```python
from build123d import *

# Parameters (mm, degrees)
SKETCH_1_W                = 83
SKETCH_1_H                = 127
EXTRUDE_1_DEPTH           = 36
SKETCH_2_W                = 77
SKETCH_2_H                = 40.7
CUT_EXTRUDE_1_DEPTH       = 22.9
SKETCH_3_W                = 77
SKETCH_3_H                = 78
CUT_EXTRUDE_4_DEPTH       = 33
SKETCH_4_W                = 31.5
SKETCH_4_H                = 25.3
EXTRUDE_2_DEPTH           = 11
SKETCH_5_W                = 25.5
SKETCH_5_H                = 23.3
CUT_EXTRUDE_5_DEPTH       = 11
CUT_EXTRUDE_6_DEPTH       = 14
CUT_EXTRUDE_6_DEPTH_BACK  = 10
SKETCH_6_R                = 1.5
SKETCH_7_R                = 2.5
CUT_EXTRUDE_7_DEPTH       = 22
CUT_EXTRUDE_8_DEPTH       = 23
CUT_EXTRUDE_8_DEPTH_BACK  = 30
SKETCH_8_R                = 2.7
CUT_EXTRUDE_9_DEPTH       = 11
CUT_EXTRUDE_9_DEPTH_BACK  = 33
SKETCH_9_W                = 12
SKETCH_9_H                = 10.9
CUT_EXTRUDE_10_DEPTH      = 14
CUT_EXTRUDE_10_DEPTH_BACK = 36
SKETCH_10_W               = 9
SKETCH_10_H               = 10.5
SKETCH_11_W               = 78
SKETCH_11_H               = 3
EXTRUDE_3_DEPTH           = 4
SKETCH_12_W               = 69
SKETCH_12_H               = 3
EXTRUDE_4_DEPTH           = 4
SKETCH_13_W               = 78
SKETCH_13_H               = 3
EXTRUDE_5_DEPTH           = 4
SKETCH_15_W               = 69
SKETCH_15_H               = 3
EXTRUDE_6_DEPTH           = 2
SKETCH_16_W               = 1.5
SKETCH_16_H               = 41.5
CUT_EXTRUDE_11_DEPTH      = 2
SKETCH_17_W               = 78.5
SKETCH_17_H               = 1.5
CUT_EXTRUDE_12_DEPTH      = 2
SKETCH_19_W               = 1.5
SKETCH_19_H               = 42.211102857
CUT_EXTRUDE_13_DEPTH      = 2
FILLET_1_R                = 2
FILLET_2_R                = 2
FILLET_3_R                = 2
FILLET_4_R                = 2
FILLET_5_R                = 2
SKETCH_20_W               = 8
SKETCH_20_H               = 10
CUT_EXTRUDE_14_DEPTH      = 2
SKETCH_21_W               = 8
SKETCH_21_H               = 10
CUT_EXTRUDE_15_DEPTH      = 2
CUT_EXTRUDE_16_DEPTH      = 102
CUT_EXTRUDE_16_DEPTH_BACK = 85
SKETCH_22_R               = 1.5
CUT_EXTRUDE_17_DEPTH      = 37
CUT_EXTRUDE_17_DEPTH_BACK = 68
SKETCH_23_R               = 1.5


with BuildPart() as part:
    # Эскиз1 → Бобышка-Вытянуть1 (new body)
    with BuildSketch(Plane(origin=(0, 0, 0), x_dir=(1, 0, 0), z_dir=(0, 1, 0))):
        with Locations((-41.5, 63.5)):
            Rectangle(SKETCH_1_W, SKETCH_1_H)
    extrude(amount=EXTRUDE_1_DEPTH)

    # Эскиз2 → Вырез-Вытянуть1 (cut)
    with BuildSketch(Plane(origin=(0, 0, 0), x_dir=(-1, 0, 0), z_dir=(0, -1, 0))):
        with Locations((41.5, 23.35)):
            Rectangle(SKETCH_2_W, SKETCH_2_H)
    extrude(amount=-CUT_EXTRUDE_1_DEPTH, mode=Mode.SUBTRACT)

    # Эскиз3 → Вырез-Вытянуть4 (cut)
    with BuildSketch(Plane(origin=(0, 36, 0), x_dir=(1, 0, 0), z_dir=(0, 1, 0))):
        with Locations((-41.5, 85)):
            Rectangle(SKETCH_3_W, SKETCH_3_H)
    extrude(amount=-CUT_EXTRUDE_4_DEPTH, mode=Mode.SUBTRACT)

    # Эскиз4 → Бобышка-Вытянуть2 (add)
    with BuildSketch(Plane(origin=(0, 3, 0), x_dir=(1, 0, 0), z_dir=(0, 1, 0))):
        with Locations((-41.5, 58.65)):
            Rectangle(SKETCH_4_W, SKETCH_4_H)
    extrude(amount=EXTRUDE_2_DEPTH)

    # Эскиз5 → Вырез-Вытянуть5 (cut)
    with BuildSketch(Plane(origin=(0, 14, 0), x_dir=(1, 0, 0), z_dir=(0, 1, 0))):
        with Locations((-41.5, 59.65)):
            Rectangle(SKETCH_5_W, SKETCH_5_H)
    extrude(amount=-CUT_EXTRUDE_5_DEPTH, mode=Mode.SUBTRACT)

    # Эскиз6 → Вырез-Вытянуть6 (cut, two sides: drawn at the far end of the back side and taken through both)
    with BuildSketch(Plane(origin=(0, 0, 0), x_dir=(0, 0, -1), z_dir=(1, 0, 0)).offset(-CUT_EXTRUDE_6_DEPTH_BACK)):
        with Locations(Location((60.742856383, 18, 0), (0, 0, 180))):
            Circle(SKETCH_6_R)
    extrude(amount=CUT_EXTRUDE_6_DEPTH + CUT_EXTRUDE_6_DEPTH_BACK, mode=Mode.SUBTRACT)

    # Эскиз7 → Вырез-Вытянуть7 (cut)
    with BuildSketch(Plane.XY.offset(-43.7)):
        with Locations((-5.5, 19.4)):
            Circle(SKETCH_7_R)
    extrude(amount=-CUT_EXTRUDE_7_DEPTH, mode=Mode.SUBTRACT)

    # Эскиз8 → Вырез-Вытянуть8 (cut, two sides: drawn at the far end of the back side and taken through both)
    with BuildSketch(Plane(origin=(0, 0, -127), x_dir=(-1, 0, 0), z_dir=(0, 0, -1)).offset(-CUT_EXTRUDE_8_DEPTH_BACK)):
        with Locations(Location((72.842031124, 26.425424665, 0), (0, 0, 180))):
            Circle(SKETCH_8_R)
    extrude(amount=CUT_EXTRUDE_8_DEPTH + CUT_EXTRUDE_8_DEPTH_BACK, mode=Mode.SUBTRACT)

    # Эскиз9 → Вырез-Вытянуть9 (cut, two sides: drawn at the far end of the back side and taken through both)
    with BuildSketch(Plane.ZY.offset(3).offset(-CUT_EXTRUDE_9_DEPTH_BACK)):
        with Locations((-87, 9.65)):
            Rectangle(SKETCH_9_W, SKETCH_9_H)
    extrude(amount=CUT_EXTRUDE_9_DEPTH + CUT_EXTRUDE_9_DEPTH_BACK, mode=Mode.SUBTRACT)

    # Эскиз10 → Вырез-Вытянуть10 (cut, two sides: drawn at the far end of the back side and taken through both)
    with BuildSketch(Plane.ZY.offset(3).offset(-CUT_EXTRUDE_10_DEPTH_BACK)):
        with Locations((-116.5, 9.35)):
            Rectangle(SKETCH_10_W, SKETCH_10_H)
    extrude(amount=CUT_EXTRUDE_10_DEPTH + CUT_EXTRUDE_10_DEPTH_BACK, mode=Mode.SUBTRACT)

    # Эскиз11 → Бобышка-Вытянуть3 (add)
    with BuildSketch(Plane.ZY.offset(3)):
        with Locations((-85, 31.5)):
            Rectangle(SKETCH_11_W, SKETCH_11_H)
    extrude(amount=EXTRUDE_3_DEPTH)

    # Эскиз12 → Бобышка-Вытянуть4 (add)
    with BuildSketch(Plane.XY.offset(-124)):
        with Locations((-41.5, 31.5)):
            Rectangle(SKETCH_12_W, SKETCH_12_H)
    extrude(amount=EXTRUDE_4_DEPTH)

    # Эскиз13 → Бобышка-Вытянуть5 (add)
    with BuildSketch(Plane(origin=(-80, 0, 0), x_dir=(0, 0, -1), z_dir=(1, 0, 0))):
        with Locations((85, 31.5)):
            Rectangle(SKETCH_13_W, SKETCH_13_H)
    extrude(amount=EXTRUDE_5_DEPTH)

    # Эскиз15 → Бобышка-Вытянуть6 (add)
    with BuildSketch(Plane(origin=(0, 0, -46), x_dir=(-1, 0, 0), z_dir=(0, 0, -1))):
        with Locations((41.5, 31.5)):
            Rectangle(SKETCH_15_W, SKETCH_15_H)
    extrude(amount=EXTRUDE_6_DEPTH)

    # Эскиз16 → Вырез-Вытянуть11 (cut)
    with BuildSketch(Plane(origin=(0, 0, 0), x_dir=(-1, 0, 0), z_dir=(0, -1, 0))):
        with Locations((2.25, 23.75)):
            Rectangle(SKETCH_16_W, SKETCH_16_H)
    extrude(amount=-CUT_EXTRUDE_11_DEPTH, mode=Mode.SUBTRACT)

    # Эскиз17 → Вырез-Вытянуть12 (cut)
    with BuildSketch(Plane.XZ):
        with Locations((-40.75, -44.45)):
            Rectangle(SKETCH_17_W, SKETCH_17_H)
    extrude(amount=-CUT_EXTRUDE_12_DEPTH, mode=Mode.SUBTRACT)

    # Эскиз19 → Вырез-Вытянуть13 (cut)
    with BuildSketch(Plane.XZ):
        with Locations((-80.75, -24.094448572)):
            Rectangle(SKETCH_19_W, SKETCH_19_H)
    extrude(amount=-CUT_EXTRUDE_13_DEPTH, mode=Mode.SUBTRACT)

    # Скругление1
    fillet_1_edges = [part.edges().sort_by_distance(p)[0] for p in [
        (-41.5, 36, -127),
    ]]
    fillet(fillet_1_edges, radius=FILLET_1_R)

    # Скругление2
    fillet_2_edges = [part.edges().sort_by_distance(p)[0] for p in [
        (-83, 36, -62.5),
        (-83, 17, -127),
        (-83, 35.414213562, -126.414213562),
    ]]
    fillet(fillet_2_edges, radius=FILLET_2_R)

    # Скругление3
    fillet_3_edges = [part.edges().sort_by_distance(p)[0] for p in [
        (-83, 17, 0),
        (-40.5, 36, 0),
        (-82.414213562, 35.414213562, 0),
    ]]
    fillet(fillet_3_edges, radius=FILLET_3_R)

    # Скругление4
    fillet_4_edges = [part.edges().sort_by_distance(p)[0] for p in [
        (0, 17, -127),
        (0, 35.414213562, -126.414213562),
        (0, 17, 0),
        (0, 36, -63.5),
        (0, 35.414213562, -0.585786438),
    ]]
    fillet(fillet_4_edges, radius=FILLET_4_R)

    # Скругление5
    # the kernel refuses this fillet: 2 mm, written as the material it takes off along each edge
    with BuildSketch(Plane(origin=(-2, 0, -125), x_dir=(1, 0, 0), z_dir=(0, 0, 1))) as fillet_5_piece_1:
        with BuildLine():
            CenterArc((2 - FILLET_5_R, FILLET_5_R), FILLET_5_R, 270, 90)
            Line((2, FILLET_5_R), (2, 0))
            Line((2, 0), (2 - FILLET_5_R, 0))
        make_face()
    revolve(axis=Axis((-2, 0, -125), (0, 1, 0)), revolution_arc=90, mode=Mode.SUBTRACT)
    with BuildSketch(Plane(origin=(0, 0, -125), x_dir=(0, 1, 0), z_dir=(0, 0, 1))) as fillet_5_piece_2:
        with BuildLine():
            CenterArc((FILLET_5_R, FILLET_5_R), FILLET_5_R, 180, 90)
            Line((0, FILLET_5_R), (0, 0))
            Line((0, 0), (FILLET_5_R, 0))
        make_face()
    extrude(amount=123, mode=Mode.SUBTRACT)
    with BuildSketch(Plane(origin=(-2, 0, -2), x_dir=(1, 0, 0), z_dir=(0, 0, -1))) as fillet_5_piece_3:
        with BuildLine():
            CenterArc((2 - FILLET_5_R, -FILLET_5_R), FILLET_5_R, 0, 90)
            Line((2, -FILLET_5_R), (2, 0))
            Line((2, 0), (2 - FILLET_5_R, 0))
        make_face()
    revolve(axis=Axis((-2, 0, -2), (0, -1, 0)), revolution_arc=90, mode=Mode.SUBTRACT)
    with BuildSketch(Plane(origin=(-2, 0, 0), x_dir=(0, 0, -1), z_dir=(-1, 0, 0)), Plane(origin=(-81, 0, -127), x_dir=(0, 0, 1), z_dir=(1, 0, 0))) as fillet_5_piece_4:
        with BuildLine():
            CenterArc((FILLET_5_R, -FILLET_5_R), FILLET_5_R, 90, 90)
            Line((0, -FILLET_5_R), (0, 0))
            Line((0, 0), (FILLET_5_R, 0))
        make_face()
    extrude(amount=79, mode=Mode.SUBTRACT)
    with BuildSketch(Plane(origin=(-81, 0, -2), x_dir=(-1, 0, 0), z_dir=(0, 0, -1))) as fillet_5_piece_5:
        with BuildLine():
            CenterArc((2 - FILLET_5_R, FILLET_5_R), FILLET_5_R, 270, 90)
            Line((2, FILLET_5_R), (2, 0))
            Line((2, 0), (2 - FILLET_5_R, 0))
        make_face()
    revolve(axis=Axis((-81, 0, -2), (0, 1, 0)), revolution_arc=90, mode=Mode.SUBTRACT)
    with BuildSketch(Plane(origin=(-83, 0, -2), x_dir=(1, 0, 0), z_dir=(0, 0, -1))) as fillet_5_piece_6:
        with BuildLine():
            CenterArc((FILLET_5_R, -FILLET_5_R), FILLET_5_R, 90, 90)
            Line((0, -FILLET_5_R), (0, 0))
            Line((0, 0), (FILLET_5_R, 0))
        make_face()
    extrude(amount=123, mode=Mode.SUBTRACT)
    with BuildSketch(Plane(origin=(-81, 0, -125), x_dir=(-1, 0, 0), z_dir=(0, 0, 1))) as fillet_5_piece_7:
        with BuildLine():
            CenterArc((2 - FILLET_5_R, -FILLET_5_R), FILLET_5_R, 0, 90)
            Line((2, -FILLET_5_R), (2, 0))
            Line((2, 0), (2 - FILLET_5_R, 0))
        make_face()
    revolve(axis=Axis((-81, 0, -125), (0, -1, 0)), revolution_arc=90, mode=Mode.SUBTRACT)

    # Эскиз20 → Вырез-Вытянуть14 (cut)
    with BuildSketch(Plane.XZ):
        with Locations((-15, -50.2)):
            Rectangle(SKETCH_20_W, SKETCH_20_H)
    extrude(amount=-CUT_EXTRUDE_14_DEPTH, mode=Mode.SUBTRACT)

    # Эскиз21 → Вырез-Вытянуть15 (cut)
    with BuildSketch(Plane.XZ):
        with Locations((-68, -50.2)):
            Rectangle(SKETCH_21_W, SKETCH_21_H)
    extrude(amount=-CUT_EXTRUDE_15_DEPTH, mode=Mode.SUBTRACT)

    # Эскиз22 → Вырез-Вытянуть16 (cut, two sides: drawn at the far end of the back side and taken through both)
    with BuildSketch(Plane.XZ.offset(-2).offset(-CUT_EXTRUDE_16_DEPTH_BACK)):
        with Locations(Location((-15, -51.2, 0), (0, 0, 270))):
            Circle(SKETCH_22_R)
    extrude(amount=CUT_EXTRUDE_16_DEPTH + CUT_EXTRUDE_16_DEPTH_BACK, mode=Mode.SUBTRACT)

    # Эскиз23 → Вырез-Вытянуть17 (cut, two sides: drawn at the far end of the back side and taken through both)
    with BuildSketch(Plane.XZ.offset(-2).offset(-CUT_EXTRUDE_17_DEPTH_BACK)):
        with Locations(Location((-68, -51.2, 0), (0, 0, 90))):
            Circle(SKETCH_23_R)
    extrude(amount=CUT_EXTRUDE_17_DEPTH + CUT_EXTRUDE_17_DEPTH_BACK, mode=Mode.SUBTRACT)


solid = part.part
```
CAD build for the part. Positions are in the model's coordinates, mm. A direction names the side the tool comes from. Give positions to 0.01 mm unless a question says otherwise; leave off trailing zeros. Order: outer loops, then holes, each group sorted by start corner. A loop starts at its lowest first (then second) coordinate and runs counter-clockwise, first axis right, second up. Notation, with made-up numbers: M -33,61.25 L -16,61.25 A29 ccw -16,95.25 Z; hole C 84,-1 d1. An arc over 180 degrees is marked long. Put each result on its own line as item: value. Start each with the question number.
(1) Saw through at C-C, the plane z = -40. Write the cut outline in (x, y).
(2) Saw through at B-B, the plane x = -5.5. Write the cut outline in (y, z), then the cut area to 3 significant figures.
(3) Drill centre lines: line 1 along Z through (x, y) = (-67.5, 9); line 2 along Z through (x, y) = (-68, 2.4); line 3 along X through (y, z) = (2.7, -51.2). Where is each one in solid material? Low to high.
(4) Which spindle directions (+Z, -Z, +X, -X, +Y, -Y) get a long thin tool onto all of the face, cutting with end or side? Do faces 1 (the flat face through (-3, 17, -84)), 2 (the flat face through (-54.25, 9, -59)), 3 (the flat face through (-1, 15.1, -87)). Say none if no direction does.
(5) Saw through at D-D, the plane x = -38. Write the cut outline in (y, z).
(6) Flat gauge pins, fed straight in: pin 1 Ø2 at (x, y) = (-66, 0.5) entering from +Z; pin 2 Ø2 at (y, z) = (0.5, -51) entering from +X; pin 3 Ø12 at (x, z) = (-60.5, -23) entering from -Y. Where does each tip first touch, or does it go through?
Check result:
1. outline: M -83,2 A2 ccw -81.5,0.06 L -81.5,2 L -80,2 L -80,22.9 L -3,22.9 L -3,2 L -1.5,2 L -1.5,0.06 A2 ccw 0,2 L 0,34 A2 ccw -2,36 L -81,36 A2 ccw -83,34 Z
2. outline: M 0,-125 A2 ccw 2,-127 L 34,-127 A2 ccw 36,-125 L 36,-124 L 33,-124 L 33,-46 L 36,-46 L 36,-2 A2 ccw 34,0 L 2,0 A2 ccw 0,-2 L 0,-3 L 22.9,-3 L 22.9,-43.7 L 21.9,-43.7 L 21.9,-46 L 30,-46 L 30,-124 L 3,-124 L 3,-46 L 16.9,-46 L 16.9,-43.7 L 2,-43.7 L 2,-45.2 L 0,-45.2 Z
2. area: 1,280 mm2
3. line 1: z = -127 to -124, -46 to -43.7, -3 to 0
3. line 2: z = -127 to -52.7, -49.7 to -43.7, -3 to 0
3. line 3: x = -83 to -69.5, -66.5 to -16.5, -13.5 to 0
4. face 1: none
4. face 2: +Y
4. face 3: +X
5. outline: M 0,-125 A2 ccw 2,-127 L 34,-127 A2 ccw 36,-125 L 36,-124 L 33,-124 L 33,-120 L 30,-120 L 30,-124 L 3,-124 L 3,-48 L 14,-48 L 14,-46 L 30,-46 L 30,-48 L 33,-48 L 33,-46 L 36,-46 L 36,-2 A2 ccw 34,0 L 2,0 A2 ccw 0,-2 L 0,-3 L 22.9,-3 L 22.9,-43.7 L 2,-43.7 L 2,-45.2 L 0,-45.2 Z
6. pin 1: stops at z = -0.06
6. pin 2: stops at x = -0.06
6. pin 3: stops at y = 22.9
